from build123d import *

# Parameters (mm, degrees)
F0_R     = 25.4
F1_DEPTH = 76.2
F2_R     = 5.08
F3_R     = 17.78
F4_DEPTH = 50.8
F5_DEPTH = 38.1


with BuildPart() as f1:
    # F0 (on Top) → F1 (new body)
    with BuildSketch(Plane.XY):
        with Locations((4.0060626761, 0)):
            Circle(F0_R)
    extrude(amount=F1_DEPTH)

    # F2
    f2_edges = [f1.edges().sort_by_distance(p)[0] for p in [
        (-21.393937, 0, 0),
    ]]
    fillet(f2_edges, radius=F2_R)

    # F3 (on face) → F4 (cut)
    with BuildSketch(Plane.XY.offset(76.2)):
        with Locations((4.0060626761, 0)):
            Circle(F3_R)
    extrude(amount=-F4_DEPTH, mode=Mode.SUBTRACT)

    # F5 (add): a face of the model
    f5_faces = [f1.faces().sort_by_distance(p)[0] for p in [
        (-20.6755168342, 0, 76.2),
    ]]
    extrude(f5_faces, amount=F5_DEPTH)


solid = f1.part
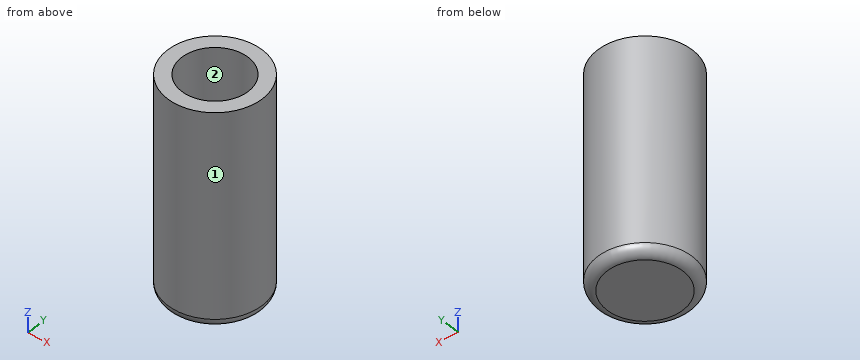
Can you work these out from the model? Positions are in its coordinate system, mm. Face numbers are marked on the shaded views. A direction names the side the tool comes from. Coordinates: 2 decimals unless noted, no trailing zeros. Loops run counter-clockwise (first coordinate to the right, second up) from the corner with the lowest first, then second, coordinate; pieces in that order, holes last. Notation, with made-up numbers: M 38,-16.75 L 55,-16.75 A21 ccw 55,22.25 Z; hole C 36.5,-2.75 d5. An arc over 180 degrees is marked long. Answer as CSV lines item,"result". Start each with the question number.
1. For the marked faces 1 and 2, which set-ups out of +Z, -Z, +X, -X, +Y, -Y let a thin tool reach every point of the face, with its end or its side?
2. For pin 1 Ø4 at (y, z) = (8, 32.5) entering from +X; pin 2 Ø8 at (x, z) = (-8.5, 45) entering from +Y; pin 3 Ø2 at (x, z) = (-13, 79.5) entering from +Y, each with a flat end and sliding along its axis, tell me the tip position at first contact or that it passes through.
3. Suppose I cut it at C-C, the plane z = 24. List the corners of the cut face in (x, y) for me.
4. Suppose I cut it at A-A, the plane y = 0. List the corners of the cut face in (x, z) for me, plus the area to 3 significant figures.
5. If I drill on probe 1 along X at (y, z) = (0.5, 107); probe 2 along Z at (x, y) = (-3, 15.5); probe 3 along X at (y, z) = (-6.5, 71), over which ranges is the centre line in solid material (lowest first)? Write a range as [from, to].
6. Suppose I cut it at B-B, the plane z = 36. List the corners of the cut face in (x, y) for me.
Output:
1,face 1,"+Z, -Z"
1,face 2,"+Z"
2,pin 1,"stops at x = 28.69"
2,pin 2,"stops at y = 23.93"
2,pin 3,"stops at y = 19.72"
3,outline,"C 4.01,0 d50.8"
4,outline,"M -21.39,5.08 A5.08 ccw -16.31,0 L 24.33,0 A5.08 ccw 29.41,5.08 L 29.41,114.3 L 21.79,114.3 L 21.79,25.4 L -13.77,25.4 L -13.77,114.3 L -21.39,114.3 Z"
4,area,"2,630 mm^2"
5,probe 1,"x = [-21.39, -13.77], [21.78, 29.4]"
5,probe 2,"z = [0, 25.4]"
5,probe 3,"x = [-20.55, -12.54], [20.56, 28.56]"
6,outline,"C 4.01,0 d50.8; hole C 4.01,0 d35.56"
